For this review, take the finished solid that the model builds, in its own axes (mm). A direction names the side the tool comes from. Give positions to 0.01 mm unless a question says otherwise; leave off trailing zeros. Loops run counter-clockwise (first coordinate to the right, second up) from the corner with the lowest first, then second, coordinate; pieces in that order, holes last. Notation, with made-up numbers: (80.5, 65.5) - (104.5, 65.5) arc R15 cw to (104.5, 84.5) - close; hole circle Ø1 at (-22, 62.5). An arc over 180 degrees is marked (long way). Put each result on its own line as item: value.
Autodesk Inventor part; units mm, degrees
ref_plane "YZ Plane" through (0, 0, 0) normal (1, 0, 0) x (0, 1, 0)
ref_plane "XZ Plane" through (0, 0, 0) normal (0, 1, 0) x (-1, 0, 0)
ref_plane "XY Plane" through (0, 0, 0) normal (0, 0, 1) x (1, 0, 0)
sketch "Sketch1" plane through (0, 0, 0) normal (0, 1, 0) x (-1, 0, 0)
  line L0 (38.1169, -26.9408) -> (65.0577, -0.0001)
  line L1 (71.6583, -6.6007) -> (33.1013, -45.1577)
  line L2 (65.0577, -0.0001) -> (71.6583, -6.6007)
  circle A0 centre (0.0001, -0.0001) radius 0.88
  line L3 (2.525, 2.4129) -> (-2.5248, 2.4129)
  line L4 (2.525, -2.4131) -> (-2.5248, -2.4131)
  arc A1 (-2.5248, 2.4129) -> (-2.5248, -2.4131) centre (0.0001, -0.0001) ccw
  arc A2 (2.525, -2.4131) -> (2.525, 2.4129) centre (0.0001, -0.0001) ccw
  line L5 (38.1169, -26.9408) -> (-0.1838, 11.3598)
  line L6 (-0.1838, 11.3598) -> (-11.8, -0.2564)
  line L7 (33.1013, -45.1577) -> (-11.8, -0.2564)
  dimension "d12" = 1.76
  dimension "d14" = 4.826
  dimension "d17" = 63.5
  dimension "d25" = 3.4925
extrude "Extrusion1" add sketch "Sketch1" along normal blind 5.08 contours L0 L2 L1 L7 L6 L5
sketch "Sketch2" plane through (0, 5.08, 0) normal (0, 1, 0) x (1, 0, 0)
  line L0 (-33.1013, 45.1577) -> (-71.6583, 6.6007)
  line L1 (-71.6583, 6.6007) -> (-65.0577, 0.0001)
  line L2 (-65.0577, 0.0001) -> (-38.1169, 26.9408)
  line L3 (-38.1169, 26.9408) -> (0.1838, -11.3598)
  line L4 (0.1838, -11.3598) -> (11.8, 0.2564)
  line L5 (11.8, 0.2564) -> (-33.1013, 45.1577)
  arc A0 (-2.525, 2.4131) -> (-2.525, -2.4129) centre (-0.0001, 0.0001) ccw
  line L6 (-2.525, 2.4131) -> (2.5248, 2.4131)
  arc A1 (2.5248, -2.4129) -> (2.5248, 2.4131) centre (-0.0001, 0.0001) ccw
  line L7 (2.5248, -2.4129) -> (-2.525, -2.4129)
  point P0 (0, 0)
properties part number "gripper (moving part"
1) Take a section at A-A on y = 4.1. State the section outline as (x, z) points (3 decimals).
Geometry check:
outline: (-71.658, -6.601) - (-33.101, -45.158) - (11.8, -0.256) - (0.184, 11.36) - (-38.117, -26.941) - (-65.058, 0) - close; hole (-2.525, -2.413) - (2.525, -2.413) arc R3.493 ccw to (2.525, 2.413) - (-2.525, 2.413) arc R3.493 ccw to start
2) Wall thickness on line 1 (X direction, y = 1.4, z = -7.5); line 2 (Z direction, x = 0.5, y = 4.5); line 3 (X direction, y = 2.75, z = -20): over which ranges is each line inside the solid? List them lowest first.
Geometry check:
line 1: x = -70.76 to -57.56, -18.68 to 4.56
line 2: z = -11.56 to -2.41, 2.41 to 11.04
line 3: x = -58.26 to -45.06, -31.18 to -7.94
3) Take a section at D-D on z = -33. State the section outline as (x, y) points.
Geometry check:
outline: (-45.26, 0) - (-20.94, 0) - (-20.94, 5.08) - (-45.26, 5.08) - close
4) Take a section at C-C on x = 1.5. State the section outline as (y, z) points, and give its area (3 significant figures).
Geometry check:
outline: (0, -10.56) - (5.08, -10.56) - (5.08, -2.41) - (0, -2.41) - close; (0, 2.41) - (5.08, 2.41) - (5.08, 10.04) - (0, 10.04) - close
area: 80.1 mm²
5) Take a section at B-B on z = -25.5. State the section outline as (x, y) points, and give its area (3 significant figures).
Geometry check:
outline: (-52.76, 0) - (-39.56, 0) - (-39.56, 5.08) - (-52.76, 5.08) - close; (-36.68, 0) - (-13.44, 0) - (-13.44, 5.08) - (-36.68, 5.08) - close
area: 185 mm²
6) Insertion check: pin 1 Ø1.5 at (y, z) = (4, 2) entering from +X; pin 2 Ø2 at (y, z) = (4, -15.5) entering from +X; pin 3 Ø2.5 at (x, y) = (0, 3) entering from -Z. Each pin has a flat end and moves straight along its axis. Give the tip position at first contact, or say it passes through.
Geometry check:
pin 1: stops at x = 10.29
pin 2: stops at x = -2.44
pin 3: stops at z = -13.31
7) For faces 1 (the face through (5.911, 2.504, 5.633)), 2 (the face through (3.492, 2.504, -0.037)), 3 (the face through (-19.235, 2.504, -8.059)), list the 3-axis set-ups (+Z, -Z, +X, -X, +Y, -Y) from which the entire face can be reached by the end or side of a thin tool; tool diameter is ignored.
Geometry check:
face 1: +Z, +X, +Y, -Y
face 2: +Y, -Y
face 3: +Z, +Y, -Y
8) Draft analysis for pull direction Z (two halves, no side actions). For faces 4 (the face through (-27, 5.08, -19)), 5 (the face through (-52.65, 2.5, -25.61)), 6 (the face through (-3.492, 2.504, 0.037)), 7 (the face through (0, 3, 2.413)), state which applies: pulls with the +Z half, pulls with the -Z half, needs draft (parallel to the pull), parting line crosses it, or undercut.
Geometry check:
face 4: needs draft
face 5: pulls with the -Z half
face 6: undercut
face 7: undercut
